Part model, mm, in its own coordinate system. Face numbers are marked on the shaded views. A direction names the side the tool comes from. Give positions to 0.01 mm unless a question says otherwise; leave off trailing zeros. Order: outer loops, then holes, each group sorted by start corner. A loop starts at its lowest first (then second) coordinate and runs counter-clockwise, first axis right, second up. Notation, with made-up numbers: M 77.25,-35 L 112.25,-35 A10 ccw 112.25,-18 Z; hole C 45.25,13 d5. An arc over 180 degrees is marked long. Return JSON: item names as keys, results as strings.
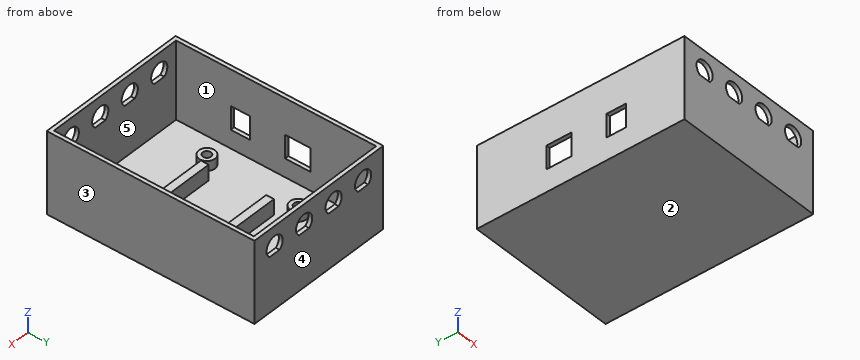
Autodesk Inventor part; units mm, degrees
ref_plane "YZ Plane" through (0, 0, 0) normal (1, 0, 0) x (0, 1, 0)
ref_plane "XZ Plane" through (0, 0, 0) normal (0, 1, 0) x (-1, 0, 0)
ref_plane "XY Plane" through (0, 0, 0) normal (0, 0, 1) x (1, 0, 0)
sketch "Sketch1" plane through (0, 0, 0) normal (0, 0, 1) x (1, 0, 0)
  line L0 (-35.3, 51.65) -> (39.3, 51.65)
  line L1 (39.3, 51.65) -> (39.3, -51.65)
  line L2 (39.3, -51.65) -> (-35.3, -51.65)
  line L3 (-35.3, -51.65) -> (-35.3, 51.65)
  line L4 (-35.3, 51.65) -> (39.3, -51.65) construction
  line L5 (39.3, 51.65) -> (-35.3, -51.65) construction
  line L6 (34.3, 26.65) -> (-34.3, 26.65) construction
  line L7 (-34.3, 26.65) -> (-34.3, -26.65) construction
  line L8 (-34.3, -26.65) -> (34.3, -26.65) construction
  line L9 (34.3, -26.65) -> (34.3, 26.65) construction
  line L10 (34.3, 26.65) -> (-34.3, -26.65) construction
  line L11 (-34.3, 26.65) -> (34.3, -26.65) construction
  circle A0 centre (-20.3, 24.05) radius 1.6 construction
  circle A1 centre (-21.6, -24.15) radius 1.6 construction
  circle A2 centre (30.5, 8.85) radius 1.6 construction
  circle A3 centre (30.5, -19.05) radius 1.6 construction
  line L12 (-37.3, 53.65) -> (41.3, 53.65)
  line L13 (41.3, 53.65) -> (41.3, -53.65)
  line L14 (41.3, -53.65) -> (-37.3, -53.65)
  line L15 (-37.3, -53.65) -> (-37.3, 53.65)
  line L16 (-37.3, 53.65) -> (41.3, -53.65) construction
  line L17 (41.3, 53.65) -> (-37.3, -53.65) construction
  line L18 (30.5, 53.65) -> (30.5, -53.65) construction
  point P0 (0, 0)
  dimension "d0" = 53.3
  dimension "d2" = 68.6
  dimension "d3" = 14
  dimension "d4" = 2.5
  dimension "d5" = 50.8
  dimension "d6" = 27.9
  dimension "d7" = 5.1
  dimension "d8" = 3.2
  dimension "d9" = 25
  dimension "d10" = 1
  dimension "d11" = 2
  dimension "d12" = 2
  dimension "d59" = 5
  dimension "d62" = 25
  dimension "d63" = 2
  dimension "d64" = 2
  dimension "d92" = 15.2
  dimension "d94" = 1.3
extrude "Extrusion1" add sketch "Sketch1" against normal blind 2 contours L0 L1 L2 L3 | L12 L13 L14 L15
extrude "Extrusion2" add sketch "Sketch1" along normal blind 40
sketch "Sketch2" plane through (0, 0, 0) normal (0, 0, 1) x (1, 0, 0)
  circle A0 centre (-21.6, -24.15) radius 1.6 construction
  circle A1 centre (-20.3, 24.05) radius 4.15
  circle A2 centre (-21.6, -24.15) radius 4.15
  circle A3 centre (30.5, -19.05) radius 4.15
  circle A4 centre (30.5, 8.85) radius 4.15
  circle A5 centre (-20.3, 24.05) radius 2.15
  circle A6 centre (30.5, 8.85) radius 2.15
  circle A7 centre (-21.6, -24.15) radius 2.15
  circle A8 centre (30.5, -19.05) radius 2.15
  point P0 (0, 0)
  dimension "d17" = 8.3
  dimension "d19" = 4.3
extrude "Extrusion3" add sketch "Sketch2" along normal blind 5
sketch "Sketch6" plane through (-37.3, 53.65, -2) normal (0, 1, 0) x (1, 0, 0)
  line L0 (78.6, -42) -> (78.6, 0)
  line L1 (0, 0) -> (78.6, 0)
  line L2 (0, 0) -> (0, -42)
  line L3 (0, -32) -> (78.6, -32) construction
  arc A0 (9.2389, -28.11) -> (15.3611, -28.11) centre (12.3, -32) ccw
  line L4 (78.6, -42) -> (0, -42)
  line L5 (12.3, -32) -> (12.3, -28.11) construction
  line L6 (9.2389, -28.11) -> (15.3611, -28.11)
  arc A1 (27.2389, -28.11) -> (33.3611, -28.11) centre (30.3, -32) ccw
  line L7 (27.2389, -28.11) -> (33.3611, -28.11)
  arc A2 (45.2389, -28.11) -> (51.3611, -28.11) centre (48.3, -32) ccw
  line L8 (45.2389, -28.11) -> (51.3611, -28.11)
  arc A3 (63.2389, -28.11) -> (69.3611, -28.11) centre (66.3, -32) ccw
  line L9 (63.2389, -28.11) -> (69.3611, -28.11)
  point P0 (37.3, -2)
  point P1 (30.3, -28.11)
  point P2 (48.3, -28.11)
  point P3 (66.3, -28.11)
  dimension "d46" = 9.9
  dimension "d54" = 12.3
  dimension "d56" = 32
  dimension "d65" = 3.89
  dimension "d68" = 18
  dimension "d73" = 12.3
extrude "Extrusion6" cut sketch "Sketch6" against normal through all contours L6 A0 | L7 A1 | L8 A2 | L9 A3
sketch "Sketch7" plane through (0, 0, 0) normal (0, 0, 1) x (1, 0, 0)
  circle A0 centre (30.5, -19.05) radius 4.15
  circle A1 centre (30.5, 8.85) radius 4.15
  line L0 (-14.3, -17.05) -> (24.5, -17.05)
  line L1 (24.5, -17.05) -> (24.5, -21.05)
  line L2 (24.5, -21.05) -> (-14.3, -21.05)
  line L3 (-14.3, -21.05) -> (-14.3, -17.05)
  line L4 (-34.3, -26.65) -> (34.3, -26.65) construction
  line L5 (34.3, 26.65) -> (-34.3, 26.65) construction
  line L6 (34.3, -26.65) -> (34.3, 26.65) construction
  line L7 (-34.3, 26.65) -> (-34.3, -26.65) construction
  line L8 (24.5, 16.65) -> (-14.3, 16.65)
  line L9 (-14.3, 16.65) -> (-14.3, 12.65)
  line L10 (-14.3, 12.65) -> (24.5, 12.65)
  line L11 (24.5, 12.65) -> (24.5, 16.65)
  point P0 (0, 0)
  point P1 (24.5, -19.05)
  dimension "d79" = 4
  dimension "d80" = 20
  dimension "d81" = 6
  dimension "d82" = 6
  dimension "d83" = 20
  dimension "d86" = 10
  dimension "d87" = 0
extrude "Extrusion7" add sketch "Sketch7" along normal blind 8 contours L0 L1 L2 L3 | L11 L10 L9 L8
sketch "Sketch4" plane through (-37.3, -53.65, -2) normal (-1, 0, 0) x (0, 0, 1)
  line L0 (11.5, 71.3) -> (23.5, 71.3)
  line L1 (23.5, 71.3) -> (23.5, 58.3)
  line L2 (23.5, 58.3) -> (11.5, 58.3)
  line L3 (11.5, 58.3) -> (11.5, 71.3)
  line L4 (11.5, 71.3) -> (23.5, 58.3) construction
  line L5 (23.5, 71.3) -> (11.5, 58.3) construction
  line L6 (23.5, 30.25) -> (11.5, 30.25)
  line L7 (11.5, 30.25) -> (11.5, 40.25)
  line L8 (11.5, 40.25) -> (23.5, 40.25)
  line L9 (23.5, 40.25) -> (23.5, 30.25)
  line L10 (23.5, 30.25) -> (11.5, 40.25) construction
  line L11 (11.5, 30.25) -> (23.5, 40.25) construction
  line L12 (2, 0) -> (2, 107.3)
  line L13 (7, 73.55) -> (7, 81.85)
  line L14 (10, 36.6) -> (10, 32.6)
  line L15 (0, 107.3) -> (42, 107.3)
  line L16 (0, 0) -> (0, 107.3)
  line L17 (42, 0) -> (0, 0)
  line L18 (42, 107.3) -> (42, 0)
  point P0 (2, 53.65)
  point P1 (2, 80.3)
  point P2 (2, 80.3)
  point P3 (2, 80.3)
  point P4 (2, 27)
  point P5 (2, 27)
  point P6 (2, 27)
  point P7 (17.5, 64.8)
  point P8 (17.5, 35.25)
  point P9 (2, 0)
  dimension "d22" = 13
  dimension "d24" = 12
  dimension "d26" = 9
  dimension "d27" = 12
  dimension "d28" = 10
  dimension "d31" = 3.25
  dimension "d88" = 1.5
  dimension "d90" = 1.5
extrude "Extrusion4" cut sketch "Sketch4" against normal up to surface (2 mm away) contours L0 L1 L2 L3 | L6 L7 L8 L9
properties part number "Arduino BNC box 1"
Q1. 3-axis set-ups, long thin cutter, end or side, ignore diameter. For the marked faces 1 and 2: which of +Z, -Z, +X, -X, +Y, -Y reach the whole face in a straight line?
Established:
{"face 1": "+Z", "face 2": "-Z, +X, -X, +Y, -Y"}
Q2. Band-saw the part on C-C (x = 22). Give the cut face in (y, z).
Established:
{"outline": "M -53.65,-2 L 53.65,-2 L 53.65,40 L 51.65,40 L 51.65,0 L 16.65,0 L 16.65,8 L 12.65,8 L 12.65,0 L -17.05,0 L -17.05,8 L -21.05,8 L -21.05,0 L -51.65,0 L -51.65,40 L -53.65,40 Z"}
Q3. Band-saw the part on B-B (z = 2.5). Give the number of separate pieces and of enclosed holes in the cut face, then the cut area to 3 significant figures.
Established:
{"separate pieces": "7", "enclosed holes": "5", "area": "1,200 mm²"}
Q4. Pin check, flat tips, straight feed: pin 1 (13 mm diameter, centred on x = -7, z = 30, fed in from +Y); pin 2 (9 mm diameter, centred on x = 31.5, y = 10, fed in from +Z); pin 3 (1.3 mm diameter, centred on x = -20.5, y = 24.5, fed in from +Z). Stop position of each tip, or through.
Established:
{"pin 1": "stops at y = 53.65", "pin 2": "stops at z = 5", "pin 3": "stops at z = 0"}
Q5. Probe line 1 along X through (y, z) = (53, 30); line 2 along X through (y, z) = (-24, 4); line 3 along X through (y, z) = (9, 0.5). List the from-to ranges inside material, lowest first.
Established:
{"line 1": "x = -37.3 to -29.95, -20.05 to -11.95, -2.05 to 6.05, 15.95 to 24.05, 33.95 to 41.3", "line 2": "x = -37.3 to -35.3, -25.75 to -23.74, -19.46 to -17.45, 39.3 to 41.3", "line 3": "x = -37.3 to -35.3, 26.35 to 28.36, 32.64 to 34.65, 39.3 to 41.3"}
Q6. Two-plate mould, pull along Y, no slides. Class the marked faces 3, 4 and 5: +Y half, -Y half, draft (parallel to the pull), parting line (faces both ways), or undercut.
Established:
{"face 3": "draft", "face 4": "+Y half", "face 5": "undercut"}
Q7. Band-saw the part on A-A (x = -7). Give the cut face in (y, z).
Established:
{"outline": "M -53.65,-2 L 53.65,-2 L 53.65,26.11 L 51.65,26.11 L 51.65,0 L 16.65,0 L 16.65,8 L 12.65,8 L 12.65,0 L -17.05,0 L -17.05,8 L -21.05,8 L -21.05,0 L -51.65,0 L -51.65,26.11 L -53.65,26.11 Z; M -53.65,34.95 L -51.65,34.95 L -51.65,40 L -53.65,40 Z; M 51.65,34.95 L 53.65,34.95 L 53.65,40 L 51.65,40 Z"}
Q8. Band-saw the part on D-D (y = 43). Give the cut face in (x, z).
Established:
{"outline": "M -37.3,-2 L 41.3,-2 L 41.3,40 L 39.3,40 L 39.3,0 L -35.3,0 L -35.3,40 L -37.3,40 Z"}
